Verification items for this drawing (mm, ordinates from the low corner). A direction names the side the tool comes from. Give positions to 0.01 mm unless a question says otherwise; leave off trailing zeros. Loops run counter-clockwise (first coordinate to the right, second up) from the corner with the lowest first, then second, coordinate; pieces in that order, holes last. Notation, with made-up numbers: M 27,32 L 85,32 A24 cw 85,68 Z; hole C 24,-22.75 d2. An arc over 180 degrees is marked long. Use a Markdown table: item, result.
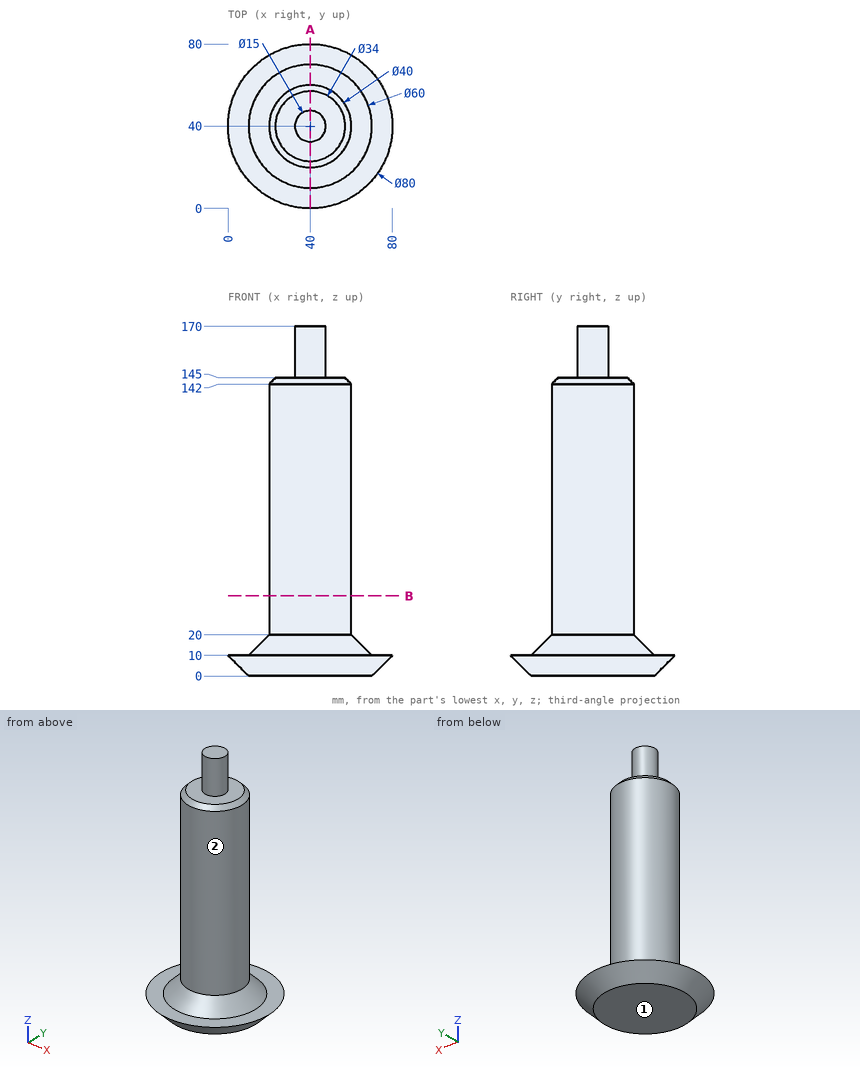
(1) Cross-section at A-A on x = 40. Record the cut outline in (y, z), then the cut area to 3 significant figures.
Results below:
| item | result |
|---|---|
| outline | M 0,10 L 10,0 L 70,0 L 80,10 L 70,10 L 60,20 L 60,142 L 57,145 L 47.5,145 L 47.5,170 L 32.5,170 L 32.5,145 L 23,145 L 20,142 L 20,20 L 10,10 Z |
| area | 6,570 mm^2 |
(2) Gauge pin test, flat ends, axial feed: P1, Ø4, axis at y = 26, z = 83.5, coming from the -X side; P2, Ø2, axis at y = 27.5, z = 39.5, coming from the -X side; P3, Ø1, axis at y = 35.5, z = 133.5, coming from the +X side; P4, Ø24, axis at x = 28, y = 50.5, coming from the +Z side. Record the tip position at first contact, or that the pin passes through.
Results below:
| item | result |
|---|---|
| P1 | x = 24 |
| P2 | x = 23.64 |
| P3 | x = 59.6 |
| P4 | z = 170 |
(3) Cross-section at B-B on z = 39. Record the cut outline in (x, y), then the cut area to 3 significant figures.
Results below:
| item | result |
|---|---|
| outline | C 40,40 d40 |
| area | 1,260 mm^2 |
(4) Material ranges on line 1 (Z direction, x = 30, y = 35); line 2 (X direction, y = 41, z = 114); line 3 (Z direction, x = 28, y = 27.5), recorded low to high.
Results below:
| item | result |
|---|---|
| line 1 | 0 to 145 |
| line 2 | 20.03 to 59.97 |
| line 3 | 0 to 144.67 |
(5) Set-up check for the marked faces 1 and 2: record each of +Z, -Z, +X, -X, +Y, -Y from which the full face is reachable in a straight line by a thin tool's end or side.
Results below:
| item | result |
|---|---|
| face 1 | -Z, +X, -X, +Y, -Y |
| face 2 | +Z |
